Source: three-view drawing plus pictorial views. Frame: mm from the lowest corner of the part. Give positions to 0.01 mm unless a question says otherwise; leave off trailing zeros. Write each loop counter-clockwise with the first axis right and the second up, starting at its lowest first coordinate (ties: lowest second). Pieces come first, ordered by that corner, then holes. Notation, with made-up numbers: M -30.5,-37 L 10.5,-37 A17 ccw 10.5,-27 Z; hole C 60.25,-1 d8. An arc over 180 degrees is marked long. Return JSON: item names as keys, results as strings.
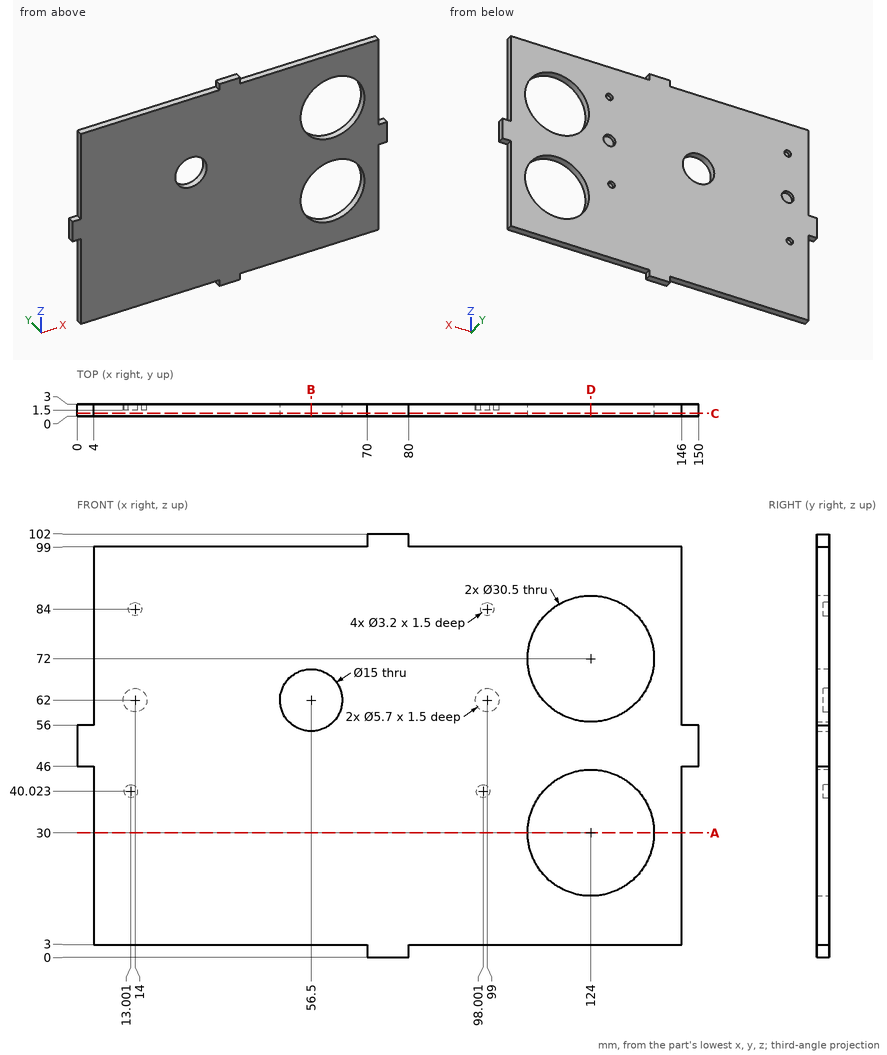
1) Contact query for flat-ended pins moving along their axis: pin 1 Ø0.9 at (y, z) = (1, 31) entering from +X; pin 2 Ø1.5 at (y, z) = (1, 2) entering from -X; pin 3 Ø1.5 at (x, y) = (1, 2) entering from +Z; pin 4 Ø10 at (x, z) = (85.5, 26.5) entering from -Y. Output: stop coordinate, or through.
Numbers:
{"pin 1": "stops at x = 146", "pin 2": "stops at x = 70", "pin 3": "stops at z = 56", "pin 4": "stops at y = 0"}
2) Line query: line 1 (Z direction, x = 125, y = 1.65); line 2 (X direction, y = 2.25, z = 73); line 3 (X direction, y = 2.5, z = 84). Output: solid intervals per line, ascending. Write a range as [from, to].
Numbers:
{"line 1": "z = [3, 14.78], [45.22, 56.78], [87.22, 99]", "line 2": "x = [4, 108.78], [139.22, 146]", "line 3": "x = [4, 12.4], [15.6, 97.4], [100.6, 114.59], [133.41, 146]"}
3) Cut plane C-C, the plane y = 0.75. Return the cut outline in (x, z), then the cut area to 3 significant figures.
Numbers:
{"outline": "M 0,46 L 4,46 L 4,3 L 70,3 L 70,0 L 80,0 L 80,3 L 146,3 L 146,46 L 150,46 L 150,56 L 146,56 L 146,99 L 80,99 L 80,102 L 70,102 L 70,99 L 4,99 L 4,56 L 0,56 Z; hole C 56.5,62 d15; hole C 124,30 d30.5; hole C 124,72 d30.5", "area": "12,100 mm²"}
4) Cut plane D-D, the plane x = 124. Return the cut outline in (y, z).
Numbers:
{"outline": "M 0,3 L 3,3 L 3,14.75 L 0,14.75 Z; M 0,45.25 L 3,45.25 L 3,56.75 L 0,56.75 Z; M 0,87.25 L 3,87.25 L 3,99 L 0,99 Z"}
5) Cut plane A-A, the plane z = 30. Return the cut outline in (x, y).
Numbers:
{"outline": "M 4,0 L 108.75,0 L 108.75,3 L 4,3 Z; M 139.25,0 L 146,0 L 146,3 L 139.25,3 Z"}
6) Cut plane B-B, the plane x = 56.5. Return the cut outline in (y, z), then the cut area to 3 significant figures.
Numbers:
{"outline": "M 0,3 L 3,3 L 3,54.5 L 0,54.5 Z; M 0,69.5 L 3,69.5 L 3,99 L 0,99 Z", "area": "243 mm²"}
